Verification items for this drawing (mm, ordinates from the low corner). Round coordinates to 2 decimals unless told otherwise and drop trailing zeros. Order: outer loops, then holes, each group sorted by start corner. A loop starts at its lowest first (then second) coordinate and runs counter-clockwise, first axis right, second up. Notation, with made-up numbers: M 6.25,71 L 43.25,71 A25 cw 43.25,108 Z; hole C 71,-12 d4. An arc over 180 degrees is marked long. One line per item, written item: value. Start each with the question number.
(1) Cross-section at B-B, the plane x = 3.5. Enter the section's corners in (y, z), and give its area (3 significant figures).
(2) Cross-section at D-D, the plane z = 3.75. Enter the section's corners in (x, y), and give its area (3 significant figures).
(3) Cross-section at C-C, the plane z = 2.5. Enter the section's corners in (x, y).
(4) Cross-section at A-A, the plane y = 5. Enter the section's corners in (x, z).
(5) Thickness scan on L1, parallel to Y at x = 8.5, z = 5; L2, parallel to Z at x = 7.5, y = 4.5. Record the ranges inside material, lowest first.
(6) Release check for a two-part mould opening along Y. For the marked faces 1, 2 and 3 record: released by +Y, released by -Y, zero draft, split by the parting line, or undercut.
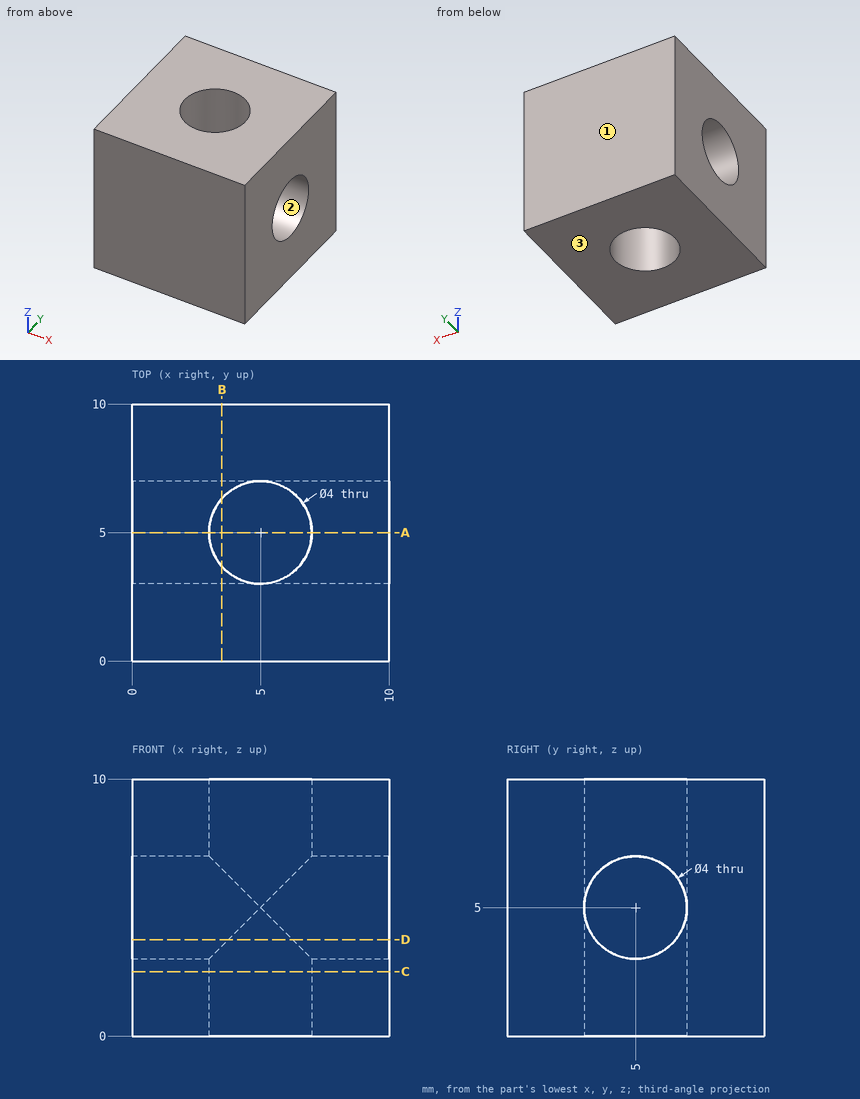
Values found:
1. outline: M 0,0 L 3.68,0 L 3.68,3.5 A2 cw 3.68,6.5 L 3.68,10 L 0,10 Z; M 6.32,0 L 10,0 L 10,10 L 6.32,10 L 6.32,6.5 A2 cw 6.32,3.5 Z
1. area: 70.7 mm^2
2. outline: M 0,0 L 10,0 L 10,3.44 L 6.25,3.44 A2 cw 3.75,3.44 L 0,3.44 Z; M 0,6.56 L 3.75,6.56 A2 cw 6.25,6.56 L 10,6.56 L 10,10 L 0,10 Z
2. area: 67.3 mm^2
3. outline: M 0,0 L 10,0 L 10,10 L 0,10 Z; hole C 5,5 d4
4. outline: M 0,0 L 3,0 L 3,3 L 0,3 Z; M 0,7 L 3,7 L 3,10 L 0,10 Z; M 7,0 L 10,0 L 10,3 L 7,3 Z; M 7,7 L 10,7 L 10,10 L 7,10 Z
5. L1: 0 to 3, 7 to 10
5. L2: 0 to 3.06, 6.94 to 10
6. face 1: released by +Y
6. face 2: undercut
6. face 3: zero draft
